```python
from build123d import *

# Parameters (mm, degrees)
F0_W     = 59
F0_H     = 84
F1_DEPTH = 10
F2_W     = 55
F2_H     = 80
F3_DEPTH = 3
F4_W     = 51
F4_H     = 76
F5_DEPTH = 5
F6_W     = 5.918054
F6_H     = 2.513148
F7_DEPTH = 0.5


with BuildPart() as f1:
    # F0 (on Top) → F1 (new body)
    with BuildSketch(Plane.XY):
        with Locations((0.888158, 11.53495)):
            Rectangle(F0_W, F0_H)
    extrude(amount=F1_DEPTH)

    # F2 (on face) → F3 (cut)
    with BuildSketch(Plane.XY.offset(10)):
        with Locations((0.888158, 11.53495)):
            Rectangle(F2_W, F2_H)
    extrude(amount=-F3_DEPTH, mode=Mode.SUBTRACT)

    # F4 (on face) → F5 (cut)
    with BuildSketch(Plane.XY.offset(7)):
        with Locations((0.888158, 11.53495)):
            Rectangle(F4_W, F4_H)
    extrude(amount=-F5_DEPTH, mode=Mode.SUBTRACT)

    # F6 (on face) → F7 (cut)
    with BuildSketch(Plane.XZ.offset(30.46505)):
        Polygon((-20.119896, 4.378146), (-20.119896, 6.891294), (-21.822348, 6.891294), (-21.822348, 8.593746), (-24.335496, 8.593746), (-24.335496, 6.891294), (-26.037948, 6.891294), (-26.037948, 4.378146), (-24.335496, 4.378146), (-24.335496, 2.675694), (-21.822348, 2.675694), (-21.822348, 4.378146), align=None)
        with Locations((24.022301, 5.63472)):
            Rectangle(F6_W, F6_H)
    extrude(amount=-F7_DEPTH, mode=Mode.SUBTRACT)


solid = f1.part
```
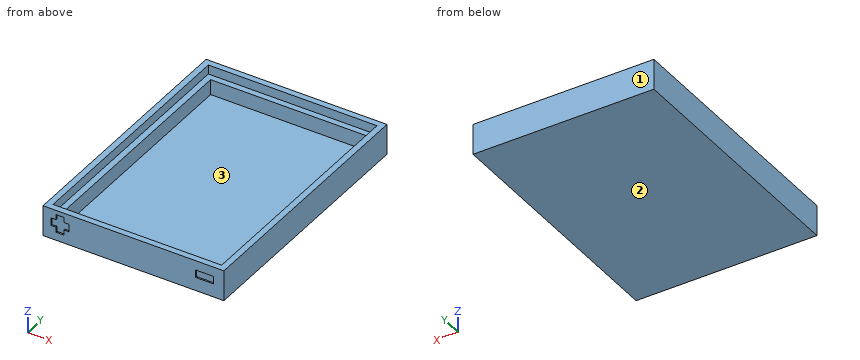
Geometry check sheet. Reference: the model listing, model coordinates, mm. Face numbers are marked on the shaded views. Coordinates: 2 decimals unless noted, no trailing zeros. Order: outer loops, then holes, each group sorted by start corner. A loop starts at its lowest first (then second) coordinate and runs counter-clockwise, first axis right, second up. Notation, with made-up numbers: M 0,26.5 L 12,26.5 A15 ccw 12,49.5 Z; hole C -26.5,-4.75 d4. An arc over 180 degrees is marked long. Answer as a JSON object with one key per item and string values.
Q1. Cross-section at C-C on y = -3. Record the cut outline in (x, z), and give its area (3 significant figures).
Results are:
{"outline": "M -28.61,0 L 30.39,0 L 30.39,10 L 28.39,10 L 28.39,7 L 26.39,7 L 26.39,2 L -24.61,2 L -24.61,7 L -26.61,7 L -26.61,10 L -28.61,10 Z", "area": "170 mm²"}
Q2. Scan lines: line 1 (Y direction, x = -3, z = 2.25); line 2 (X direction, y = 29.5, z = 8); line 3 (X direction, y = 38, z = 4.25). Record each from-to range of solid material in increasing order.
Results are:
{"line 1": "y = -30.47 to -26.47, 49.53 to 53.53", "line 2": "x = -28.61 to -26.61, 28.39 to 30.39", "line 3": "x = -28.61 to -24.61, 26.39 to 30.39"}
Q3. Cross-section at B-B on x = -2. Record the cut outline in (y, z).
Results are:
{"outline": "M -30.47,0 L 53.53,0 L 53.53,10 L 51.53,10 L 51.53,7 L 49.53,7 L 49.53,2 L -26.47,2 L -26.47,7 L -28.47,7 L -28.47,10 L -30.47,10 Z"}
Q4. Cross-section at A-A on z = 6. Record the cut outline in (x, y), and give its area (3 significant figures).
Results are:
{"outline": "M -28.61,-30.47 L -26.04,-30.47 L -26.04,-29.97 L -20.12,-29.97 L -20.12,-30.47 L 21.06,-30.47 L 21.06,-29.97 L 26.98,-29.97 L 26.98,-30.47 L 30.39,-30.47 L 30.39,53.53 L -28.61,53.53 Z; hole M -24.61,-26.47 L 26.39,-26.47 L 26.39,49.53 L -24.61,49.53 Z", "area": "1,070 mm²"}
Q5. Release check for a two-part mould opening along Y. For the marked faces 1, 2 and 3 record: released by +Y, released by -Y, zero draft, split by the parting line, or undercut.
Results are:
{"face 1": "released by +Y", "face 2": "zero draft", "face 3": "undercut"}
